Geometry: see drawing. Coordinates: mm, zero at the bounding-box minimum. A direction names the side the tool comes from. Coordinates: 2 decimals unless noted, no trailing zeros. Write each loop counter-clockwise with the first axis right and the second up, starting at its lowest first coordinate (ties: lowest second). Pieces come first, ordered by that corner, then holes. Notation, with made-up numbers: M 9,49 L 46,49 A24 cw 46,86 Z; hole C 36.5,26.25 d11. An arc over 180 degrees is marked long. Answer as CSV lines item,"result". Start each with the question number.
1. Section B-B on z = 3.5. Return the cut outline in (x, y).
2. Section C-C on x = 28.5. Return the cut outline in (y, z), plus the area to 3 significant figures.
3. Contact query for flat-ended pins moving along their axis: pin 1 Ø10 at (x, y) = (27.5, 19) entering from +Z; pin 2 Ø4 at (x, z) = (55, 19) entering from -Y; pin 3 Ø0.5 at (x, y) = (34.5, 63.5) entering from +Z. Output: stop coordinate, or through.
4. Mould query, pull axis X, two halves, no side actions, for the marked faces 3, 4, 5 and 6. Classes: pulls with the +X half, pulls with the -X half, needs draft (parallel to the pull), parting line crosses it, or undercut.
5. Reachability of the marked faces 1 and 2 from +Z, -Z, +X, -X, +Y, -Y: full face, straight path, thin tool, end or side. Return the list, or none.
6. Section D-D on y = 29. Return the cut outline in (x, z).
7. Line query: probe 1 along X at (y, z) = (17, 9.25); probe 2 along Y at (x, z) = (55, 6.75); probe 3 along Z at (x, y) = (7, 34). Output: solid intervals per line, ascending. Write a range as [from, to].
8. Section A-A on z = 8. Return the cut outline in (x, y).
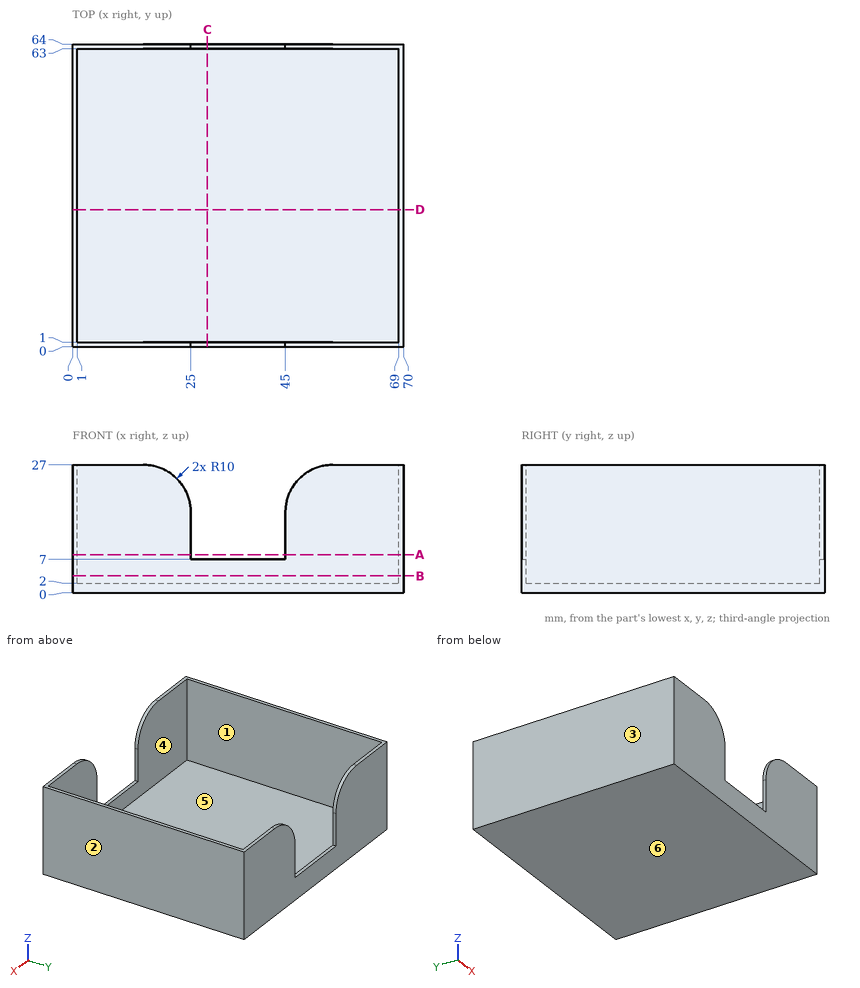
Values:
1,outline,"M 0,0 L 70,0 L 70,64 L 0,64 Z; hole M 1,1 L 69,1 L 69,63 L 1,63 Z"
2,outline,"M 0,0 L 64,0 L 64,7 L 63,7 L 63,2 L 1,2 L 1,7 L 0,7 Z"
2,area,"138 mm²"
3,pin 1,"z = 2"
3,pin 2,"y = 0"
3,pin 3,"z = 7"
4,face 3,"pulls with the -X half"
4,face 4,"undercut"
4,face 5,"undercut"
4,face 6,"needs draft"
5,face 1,"+Z"
5,face 2,"+Z, -Z, +X, +Y, -Y"
6,outline,"M 0,0 L 70,0 L 70,27 L 69,27 L 69,2 L 1,2 L 1,27 L 0,27 Z"
7,probe 1,"[0, 1], [69, 70]"
7,probe 2,"[0, 1], [63, 64]"
7,probe 3,"[0, 2]"
8,outline,"M 0,0 L 25,0 L 25,1 L 1,1 L 1,63 L 25,63 L 25,64 L 0,64 Z; M 45,0 L 70,0 L 70,64 L 45,64 L 45,63 L 69,63 L 69,1 L 45,1 Z"
